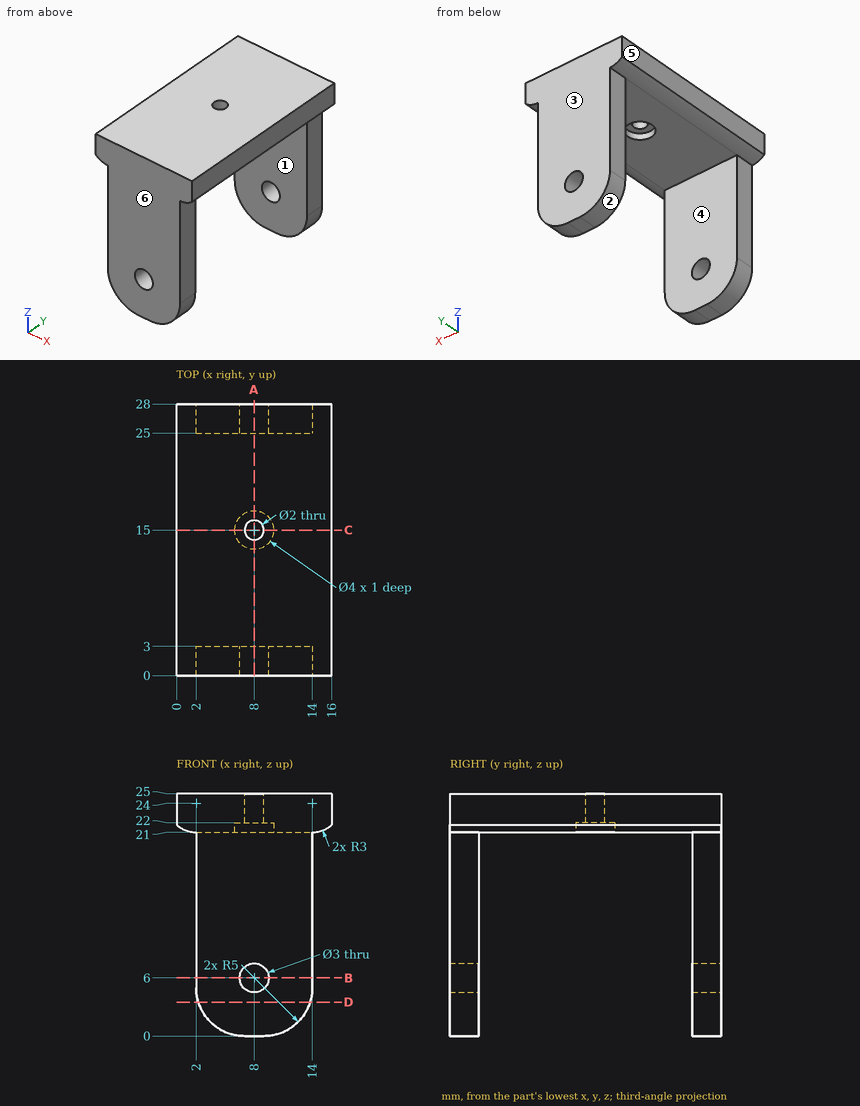
Could you check a few things on this drawing? It's one solid part, dimensions in mm from its lowest x, y, z. A direction names the side the tool comes from. Coordinates: 2 decimals unless noted, no trailing zeros. Write each loop counter-clockwise with the first axis right and the second up, starting at its lowest first coordinate (ties: lowest second). Pieces come first, ordered by that corner, then holes.
Q1. If we mould it in two halves opening along Y, with no side actions, what happens to the marked faces 3, 4, 5 and 6? For each: +Y half, -Y half, draft (parallel to the pull), parting line (faces both ways), or undercut.
Results found:
face 3: +Y half
face 4: undercut
face 5: draft
face 6: -Y half
Q2. Imagine slicing it at B-B, the plane z = 6. List the corners of the cut face in (x, y) for me.
Results found:
outline: (2, 0) - (6.5, 0) - (6.5, 3) - (2, 3) - close; (2, 25) - (6.5, 25) - (6.5, 28) - (2, 28) - close; (9.5, 0) - (14, 0) - (14, 3) - (9.5, 3) - close; (9.5, 25) - (14, 25) - (14, 28) - (9.5, 28) - close
Q3. Imagine slicing it at A-A, the plane x = 8. List the corners of the cut face in (y, z) for me.
Results found:
outline: (0, 0) - (3, 0) - (3, 4.5) - (0, 4.5) - close; (0, 7.5) - (3, 7.5) - (3, 21) - (13, 21) - (13, 22) - (14, 22) - (14, 25) - (0, 25) - close; (16, 22) - (17, 22) - (17, 21) - (25, 21) - (25, 7.5) - (28, 7.5) - (28, 25) - (16, 25) - close; (25, 0) - (28, 0) - (28, 4.5) - (25, 4.5) - close
Q4. For P1, Ø9.5, axis at x = 8.5, y = 16.5, coming from the -Z side; P2, Ø1.5, axis at y = 1, z = 17, coming from the +X side; P3, Ø1.5, axis at y = 1.5, z = 15, coming from the -X side, each with a flat end and sliding along its axis, tell me the tip position at first contact or that it passes through.
Results found:
P1: stops at z = 21
P2: stops at x = 14
P3: stops at x = 2
Q5. Please list where these lines run through material, in increasing order: L1, parallel to Y at x = 7.5, z = 3.25; L2, parallel to Y at x = 8, z = 21.7; L3, parallel to Z at x = 8, y = 27.05.
Results found:
L1: y = 0 to 3, 25 to 28
L2: y = 0 to 13, 17 to 28
L3: z = 0 to 4.5, 7.5 to 25
Q6. Which directions (+Z, -Z, +X, -X, +Y, -Y) give clear straight access to the entire face, cutting with the end or side of a thin tool? Please do the marked faces 1 and 2.
Results found:
face 1: -Z, +X, -X
face 2: -Z, -X, +Y, -Y
Q7. Imagine slicing it at C-C, the plane y = 15. List the corners of the cut face in (x, z) for me.
Results found:
outline: (0, 21.76) arc R3 ccw to (2, 21) - (6, 21) - (6, 22) - (7, 22) - (7, 25) - (0, 25) - close; (9, 22) - (10, 22) - (10, 21) - (14, 21) arc R3 ccw to (16, 21.76) - (16, 25) - (9, 25) - close
Q8. Imagine slicing it at D-D, the plane z = 3.5. List the corners of the cut face in (x, y) for me, plus the area to 3 significant figures.
Results found:
outline: (2.23, 0) - (13.77, 0) - (13.77, 3) - (2.23, 3) - close; (2.23, 25) - (13.77, 25) - (13.77, 28) - (2.23, 28) - close
area: 69.2 mm2
